The figure shows three views and two pictorial views of one solid part (mm, origin at its lowest corner). Answer the questions. A direction names the side the tool comes from. Coordinates: 2 decimals unless noted, no trailing zeros. Loops run counter-clockwise (first coordinate to the right, second up) from the corner with the lowest first, then second, coordinate; pieces in that order, holes last. Notation, with made-up numbers: M 58.25,54.5 L 113.25,54.5 A31 ccw 113.25,86.5 Z; hole C 59,80.5 d9. An arc over 180 degrees is marked long. Answer as a JSON object with one key per item and string values. Group by question number.
1. A cutting plane is placed at D-D on z = 23.25. Give the vertices of the cut face in (x, y) (3 decimals).
2. For the marked faces 1 and 2, determine the directions among +Z, -Z, +X, -X, +Y, -Y from which every point of the face is accessible in a straight line to the end or side of a thin tool.
3. Determine the mould class of the marked faces 3, 4, 5 and 6 for opening direction X: released by +X, released by -X, zero draft, split by the parting line, or undercut.
4. Given pin 1 (5.5 mm diameter, centred on y = 39.6, z = 15.88, fed in from +X); pin 2 (3 mm diameter, centred on x = 18.5, y = 35, fed in from +Z); pin 3 (4 mm diameter, centred on x = 69.85, y = 69.85, fed in from -Z), each flat-ended and moving along its own axis, determine where each tip first touches the part or whether it passes through.
5. Straight lines are drawn through the part: L1, parallel to Y at x = 69.5, z = 12; L2, parallel to X at y = 32, z = 8.5; L3, parallel to X at y = 7, z = 6.75. For each, find the intervals that lie inside material, in ascending order.
6. A cutting plane is placed at C-C on x = 69.85. Give the vertices of the cut face in (y, z) (3 decimals).
7. A cutting plane is placed at A-A on x = 6.35. Give the vertices of the cut face in (y, z) (3 decimals), and give its area (3 significant figures).
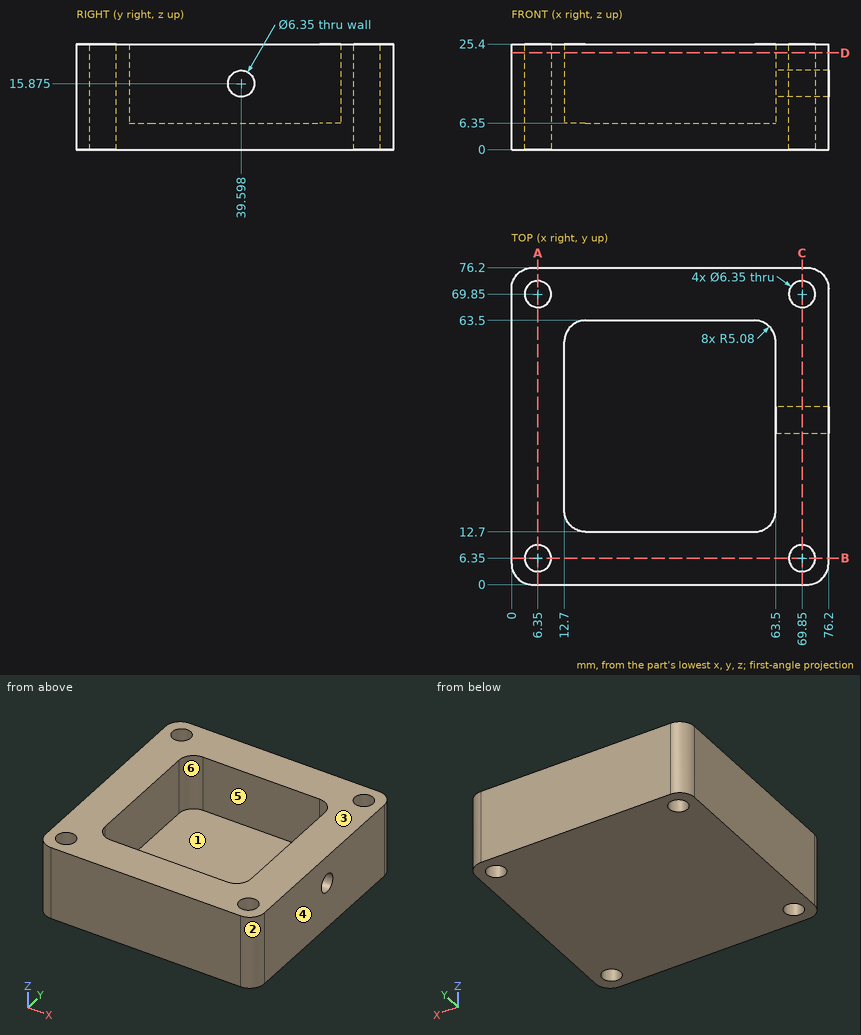
From the geometry:
{
 "1": {"outline": "M 0,5.08 A5.08 ccw 5.08,0 L 71.12,0 A5.08 ccw 76.2,5.08 L 76.2,71.12 A5.08 ccw 71.12,76.2 L 5.08,76.2 A5.08 ccw 0,71.12 Z; hole C 6.35,6.35 d6.35; hole C 6.35,69.85 d6.35; hole M 12.7,17.78 A5.08 ccw 17.78,12.7 L 58.42,12.7 A5.08 ccw 63.5,17.78 L 63.5,58.42 A5.08 ccw 58.42,63.5 L 17.78,63.5 A5.08 ccw 12.7,58.42 Z; hole C 69.85,6.35 d6.35; hole C 69.85,69.85 d6.35"},
 "2": {"face 1": "+Z", "face 2": "+Z, -Z, +X, -Y"},
 "3": {"face 3": "zero draft", "face 4": "released by +X", "face 5": "undercut", "face 6": "undercut"},
 "4": {"pin 1": "stops at x = 12.7", "pin 2": "stops at z = 6.35", "pin 3": "passes through"},
 "5": {"L1": "y = 0 to 3.19, 9.51 to 66.69, 73.01 to 76.2", "L2": "x = 0 to 12.7, 63.5 to 76.2", "L3": "x = 0 to 3.24, 9.46 to 66.74, 72.96 to 76.2"},
 "6": {"outline": "M 0,0 L 3.175,0 L 3.175,25.4 L 0,25.4 Z; M 9.525,0 L 66.675,0 L 66.675,25.4 L 9.525,25.4 Z; M 73.025,0 L 76.2,0 L 76.2,25.4 L 73.025,25.4 Z; hole C 39.598,15.875 d6.35"},
 "7": {"outline": "M 0,0 L 3.175,0 L 3.175,25.4 L 0,25.4 Z; M 9.525,0 L 66.675,0 L 66.675,25.4 L 9.525,25.4 Z; M 73.025,0 L 76.2,0 L 76.2,25.4 L 73.025,25.4 Z", "area": "1,610 mm²"}
}
